Build history of the part. All positions in model axes, mm. Give positions to 0.01 mm unless a question says otherwise; leave off trailing zeros. Loops run counter-clockwise (first coordinate to the right, second up) from the corner with the lowest first, then second, coordinate; pieces in that order, holes last.
1) Band-saw the part on B-B on x = -100.5. List the corners of the cut face in (y, z).
2) Flat gauge pins, fed straight in: P1, Ø2.5, axis at y = 5.5, z = 57.5, coming from the -X side; P2, Ø4, axis at y = 1.5, z = -78, coming from the +X side; P3, Ø4, axis at x = 6, y = 3, coming from the +Z side; P4, Ø8, axis at x = -36.5, z = -1, coming from the -Y side. Where does each tip first touch, or does it go through?
3) Band-saw the part on C-C on z = -105. List the corners of the cut face in (x, y), then the cut area to 3 significant figures.
4) Band-saw the part on A-A on y = 6. State how many separate pieces and enclosed holes the cut face has, then the cut area to 3 significant figures.
5) Wall check: line 1 (X direction, y = 5, z = 59); line 2 (Z direction, x = -61.5, y = 3); line 3 (Z direction, x = -4, y = 4.5). Give the ranges that are in metal, low to high.
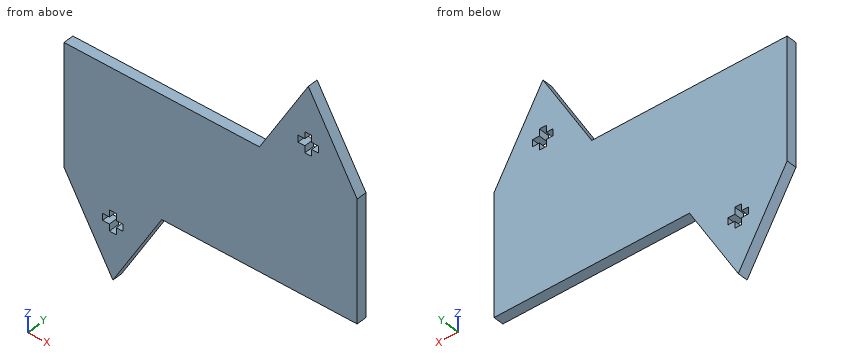
```python
from build123d import *

# Parameters (mm, degrees)
BOSS_EXTRUDE1_DEPTH = 7.62


with BuildPart() as part:
    # Sketch1 → Boss-Extrude1 (new body)
    with BuildSketch(Plane(origin=(0, 0, 0), x_dir=(1, 0, 0), z_dir=(0, 1, 0))):
        Polygon((-108.230047059, 57.852952941), (36.189952941, 57.852952941), (36.189952941, -32.306887059), (0.084952941, -94.842581466), (-36.020047059, -32.306887059), (-180.440047059, -32.306887059), (-180.440047059, 57.852952941), (-144.335047059, 120.388647348), align=None)
        Polygon((7.704952941, -50.611397059), (7.704952941, -55.691397059), (2.624952941, -55.691397059), (2.624952941, -60.771397059), (-2.455047059, -60.771397059), (-2.455047059, -55.691397059), (-7.535047059, -55.691397059), (-7.535047059, -50.611397059), (-2.455047059, -50.611397059), (-2.455047059, -45.531397059), (2.624952941, -45.531397059), (2.624952941, -50.611397059), align=None, mode=Mode.SUBTRACT)
        Polygon((-146.875047059, 81.237462941), (-151.955047059, 81.237462941), (-151.955047059, 76.157462941), (-146.875047059, 76.157462941), (-146.875047059, 71.077462941), (-141.795047059, 71.077462941), (-141.795047059, 76.157462941), (-136.715047059, 76.157462941), (-136.715047059, 81.237462941), (-141.795047059, 81.237462941), (-141.795047059, 86.317462941), (-146.875047059, 86.317462941), align=None, mode=Mode.SUBTRACT)
    extrude(amount=BOSS_EXTRUDE1_DEPTH)


solid = part.part
```
Findings below:
1. outline: (0, -57.85) - (7.62, -57.85) - (7.62, 32.31) - (0, 32.31) - close
2. P1: stops at x = -22.2
2. P2: stops at x = -118.71
2. P3: stops at z = 88.06
2. P4: stops at y = 0
3. outline: (-153.22, 0) - (-135.45, 0) - (-135.45, 7.62) - (-153.22, 7.62) - close
3. area: 135 mm2
4. separate pieces: 1
4. enclosed holes: 2
4. area: 23,800 mm2
5. line 1: x = -20.61 to -2.46, 2.62 to 20.78
5. line 2: z = -57.85 to 32.31
5. line 3: z = -57.85 to 50.61, 55.69 to 87.77
